Work out the finished part from the listing and answer in its coordinate system (mm). A direction names the side the tool comes from. Round coordinates to 2 decimals unless told otherwise and drop trailing zeros. Loops run counter-clockwise (first coordinate to the right, second up) from the corner with the lowest first, then second, coordinate; pieces in that order, holes last. Notation, with made-up numbers: (74, -29) - (86, -29) arc R23 cw to (86, 6) - close; hole circle Ø6 at (61, -18.5). An arc over 180 degrees is marked (long way). Answer as CSV lines item,"result". Start each with the question number.
Q1. Section C-C on z = 12 is taken. Write down the section's boundary in (x, y).
Q2. For faces 4 (the face through (-17.584, 1, 1)), 5 (the face through (0, 37, 38.735)), 6 (the face through (0, 37, 36.195)), determine the directions among +Z, -Z, +X, -X, +Y, -Y from which every point of the face is accessible in a straight line to the end or side of a thin tool.
Q3. The mould has two halves that part along X. Classify faces 1 (the face through (-25.489, 11.153, 0.542)), 2 (the face through (23.315, 12.468, 0.507)), 3 (the face through (-18, 0, 0)): +X half, -X half, draft (parallel to the pull), parting line (faces both ways), or undercut.
Q4. Section D-D on x = 23.5 is taken. Write down the section's boundary in (y, z) (3 decimals), then the cut area to 3 significant figures.
Q5. Straight lines are drawn through the part: L1, parallel to Z at x = -24.5, y = 22 (3 decimals); L2, parallel to X at y = 33, z = -24; L3, parallel to X at y = 15, z = 22. For each, find the intervals that lie inside material, in ascending order. Write a range as [from, to].
Q6. Section A-A on y = 54.5 is taken. Write down the section's boundary in (x, z) (3 decimals), then the cut area to 3 significant figures.
Q7. Each of these flat-tipped pins is pushed along its axis until it touches: pin 1 Ø8 at (y, z) = (7.5, 13) entering from -X; pin 2 Ø6 at (y, z) = (16.5, -25.5) entering from -X; pin 3 Ø10 at (x, z) = (-23.5, -3) entering from -Y; pin 4 Ø1.3 at (y, z) = (1, 17.5) entering from -X. Where does it stop, or does it pass through?
Q8. Section B-B on x = -4.5 is taken. Write down the section's boundary in (y, z) (3 decimals), then the cut area to 3 significant figures.
```python
from build123d import *

# Parameters (mm, degrees)
BOSS_EXTRUDE1_DEPTH = 38.735
SHELL1_T            = -2.54
SKETCH4_W           = 35.167060632
SKETCH4_H           = 72.39
CUT_EXTRUDE1_DEPTH  = 87.281603677


with BuildPart() as part:
    # Sketch1 → Boss-Extrude1 (new, symmetric)
    with BuildSketch(Plane.XY):
        Polygon((-19.05, 0), (19.05, 0), (31.75, 21.997045256), (31.75, 72.797045256), (-31.75, 72.797045256), (-31.75, 21.997045256), align=None)
    extrude(amount=BOSS_EXTRUDE1_DEPTH, both=True)

    # Shell1
    shell1_openings = [part.faces().sort_by_distance(p)[0] for p in [
        (0, 72.797045256, 0),
    ]]
    offset(amount=SHELL1_T, openings=shell1_openings, kind=Kind.INTERSECTION)

    # Sketch4 → Cut-Extrude1 (cut, through all)
    with BuildSketch(Plane(origin=(0, 2.54, 0), x_dir=(1, 0, 0), z_dir=(0, 1, 0))):
        Rectangle(SKETCH4_W, SKETCH4_H)
    extrude(amount=-CUT_EXTRUDE1_DEPTH, mode=Mode.SUBTRACT)


solid = part.part
```
Findings:
1,outline,"(-31.75, 22) - (-19.05, 0) - (-17.58, 0) - (-17.58, 2.54) - (-29.21, 22.68) - (-29.21, 72.8) - (-31.75, 72.8) - close; (17.58, 0) - (19.05, 0) - (31.75, 22) - (31.75, 72.8) - (29.21, 72.8) - (29.21, 22.68) - (17.58, 2.54) - close"
2,face 4,"+Y, -Y"
2,face 5,"+Z, +X, -X, +Y, -Y"
2,face 6,"+Y"
3,face 1,"-X half"
3,face 2,"undercut"
3,face 3,"draft"
4,outline,"(7.708, -38.735) - (72.797, -38.735) - (72.797, -36.195) - (12.788, -36.195) - (12.788, 36.195) - (72.797, 36.195) - (72.797, 38.735) - (7.708, 38.735) - close"
4,area,"698 mm^2"
5,L1,"z = [-38.735, -36.195], [36.195, 38.735]"
5,L2,"x = [-31.75, -29.21], [29.21, 31.75]"
5,L3,"x = [-27.71, -24.78], [24.78, 27.71]"
6,outline,"(-31.75, -38.735) - (31.75, -38.735) - (31.75, 38.735) - (-31.75, 38.735) - close; hole (-29.21, -36.195) - (29.21, -36.195) - (29.21, 36.195) - (-29.21, 36.195) - close"
6,area,"690 mm^2"
7,pin 1,"stops at x = -25.69"
7,pin 2,"stops at x = -30.31"
7,pin 3,"stops at y = 0"
7,pin 4,"stops at x = -20"
8,outline,"(0, -38.735) - (72.797, -38.735) - (72.797, -36.195) - (0, -36.195) - close; (0, 36.195) - (72.797, 36.195) - (72.797, 38.735) - (0, 38.735) - close"
8,area,"370 mm^2"
